Geometry check sheet. Reference: drawing and pictorial views, mm from the part's lowest x, y, z. Round coordinates to 2 decimals unless told otherwise and drop trailing zeros. Write each loop counter-clockwise with the first axis right and the second up, starting at its lowest first coordinate (ties: lowest second). Pieces come first, ordered by that corner, then holes. Notation, with made-up numbers: (-6, 70.25) -> (11, 70.25) arc R31 ccw to (11, 106.25) -> close; hole circle Ø3 at (-3, 32.25). An arc over 180 degrees is marked (long way). Answer as a JSON object with one key per item and string values. Group by question number.
(1) Sectioned sample at D-D on y = 1.5. Record the cut outline in (x, z), and give its area (3 significant figures).
(2) Sectioned sample at A-A on x = 11.44. Record the cut outline in (y, z), and give its area (3 significant figures).
(3) Scan lines: L1, parallel to Y at x = 11.44, z = 1.1; L2, parallel to Y at x = 15.24, z = 0.45; L3, parallel to Y at x = 3.7, z = 0.4. Record each from-to range of solid material in increasing order. Write a range as from..to.
(4) Sectioned sample at B-B on z = 1.1. Record the cut outline in (x, y).
(5) Draft check along X on the marked faces 1, 2 and 3. Enter one of: released by +X, released by -X, zero draft, split by the parting line, or undercut.
(6) Sectioned sample at C-C on x = 15. Record the cut outline in (y, z), and give its area (3 significant figures).
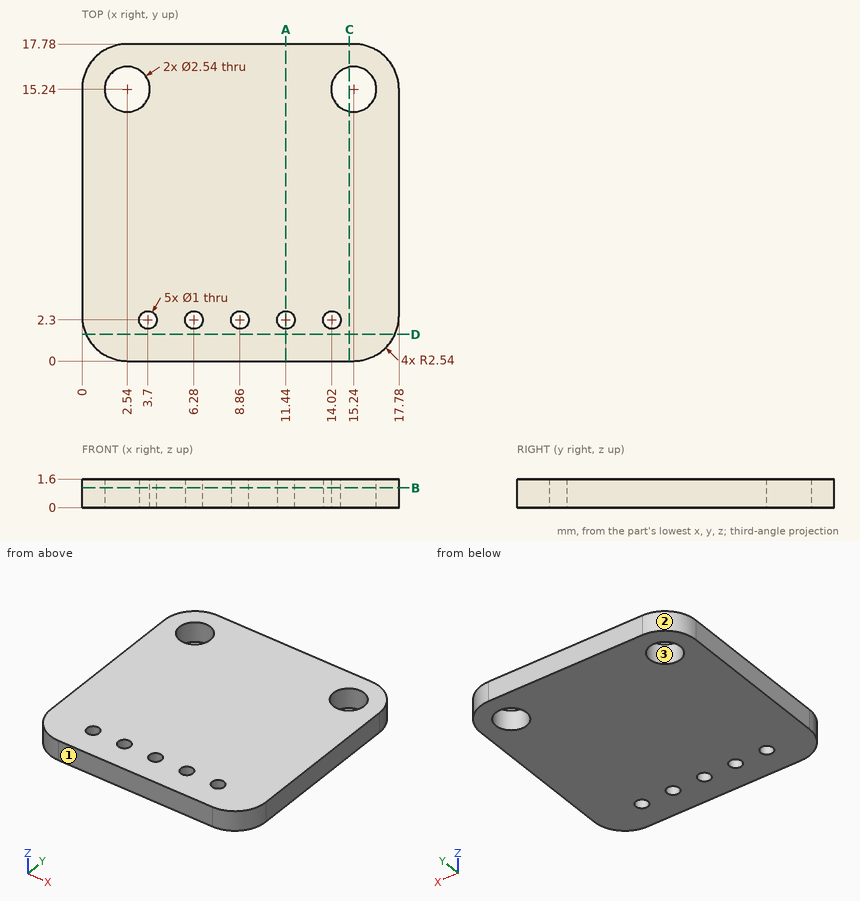
Computed values:
{
 "1": {"outline": "(0.22, 0) -> (17.56, 0) -> (17.56, 1.6) -> (0.22, 1.6) -> close", "area": "27.7 mm2"},
 "2": {"outline": "(0, 0) -> (1.8, 0) -> (1.8, 1.6) -> (0, 1.6) -> close; (2.8, 0) -> (17.78, 0) -> (17.78, 1.6) -> (2.8, 1.6) -> close", "area": "26.8 mm2"},
 "3": {"L1": "0..1.8, 2.8..17.78", "L2": "0..13.97, 16.51..17.78", "L3": "0..1.8, 2.8..14.72, 15.76..17.78"},
 "4": {"outline": "(0, 2.54) arc R2.54 ccw to (2.54, 0) -> (15.24, 0) arc R2.54 ccw to (17.78, 2.54) -> (17.78, 15.24) arc R2.54 ccw to (15.24, 17.78) -> (2.54, 17.78) arc R2.54 ccw to (0, 15.24) -> close; hole circle Ø2.54 at (2.54, 15.24); hole circle Ø1 at (3.7, 2.3); hole circle Ø1 at (6.28, 2.3); hole circle Ø1 at (8.86, 2.3); hole circle Ø1 at (11.44, 2.3); hole circle Ø1 at (14.02, 2.3); hole circle Ø2.54 at (15.24, 15.24)"},
 "5": {"face 1": "zero draft", "face 2": "released by -X", "face 3": "undercut"},
 "6": {"outline": "(0, 0) -> (13.99, 0) -> (13.99, 1.6) -> (0, 1.6) -> close; (16.49, 0) -> (17.78, 0) -> (17.78, 1.6) -> (16.49, 1.6) -> close", "area": "24.5 mm2"}
}
